CAD build for the part. Positions are in the model's coordinates, mm. A direction names the side the tool comes from. Give positions to 0.01 mm unless a question says otherwise; leave off trailing zeros. Loops run counter-clockwise (first coordinate to the right, second up) from the corner with the lowest first, then second, coordinate; pieces in that order, holes last. Notation, with made-up numbers: (2, 63.25) -> (47, 63.25) arc R9 cw to (47, 79.25) -> close; hole circle Ø1 at (88, -39). An arc over 180 degrees is marked (long way). Use one line per item in the form item = value.
```python
from build123d import *

# Parameters (mm, degrees)
F0_R     = 7.62
F1_DEPTH = 50.8
F2_R     = 1.905
F3_DEPTH = 5.715
F4_W     = 3.81
F4_H     = 7.62
F5_DEPTH = 11.431


with BuildPart() as f1:
    # F0 (on Right) → F1 (new body, symmetric)
    with BuildSketch(Plane.YZ):
        Circle(F0_R)
    extrude(amount=F1_DEPTH, both=True)

    # F2 (on Front) → F3 (join, symmetric)
    with BuildSketch(Plane.XZ):
        with BuildLine():
            Line((50.8, 3.81), (50.8, 0))
            Line((50.8, 0), (50.8, -3.81))
            Line((50.8, -3.81), (58.42, -3.81))
            ThreePointArc((58.42, -3.81), (62.23, 0), (58.42, 3.81))
            Line((58.42, 3.81), (50.8, 3.81))
        make_face()
        with Locations((58.42, 0)):
            Circle(F2_R, mode=Mode.SUBTRACT)
    extrude(amount=F3_DEPTH, both=True)

    # F4 (on face) → F5 (cut, through all)
    with BuildSketch(Plane.YZ.offset(50.8)):
        Rectangle(F4_W, F4_H)
    extrude(amount=F5_DEPTH, mode=Mode.SUBTRACT)

    # F6: F1 across plane


with BuildPart() as f1_1:
    add(f1.part)
    add(f1.part.mirror(Plane.YZ))


solid = f1_1.part
```
1. Drop flat-ended pins along their axis: P1, Ø6, axis at x = -58.42, z = 0, coming from the -Y side (3 decimals); P2, Ø5, axis at x = -3, z = 3.5, coming from the -Y side; P3, Ø6, axis at x = -8.5, y = -1, coming from the -Z side; P4, Ø1.1, axis at x = -55, y = 4.5, coming from the -Z side. Give the stop position or say it passes through.
Result sheet:
P1 = -5.715
P2 = -7.55
P3 = -7.62
P4 = -3.81
2. Tool access for faces 4 (the flat face through (-55, 4, 3.81)), 5 (the flat face through (-55, -4, -3.81)), 6 (the flat face through (55, 4, -3.81)), 7 (the flat face through (-55, -5.715, 0)), 8 (the flat face through (55, 4, 3.81)): list every direction of +Z, -Z, +X, -X, +Y, -Y with a clear straight run to the whole face (end or side of a thin tool).
Result sheet:
face_4 = +Z, -X, +Y, -Y
face_5 = -Z, -X, +Y, -Y
face_6 = -Z, +X, +Y, -Y
face_7 = +Z, -Z, -X, -Y
face_8 = +Z, +X, +Y, -Y
3. Cut at A-A, the plane y = -4.5. Write the cut outline in (x, z) (3 decimals), then the cut area to 3 significant figures.
Result sheet:
outline = (-58.42, -3.81) -> (-50.8, -3.81) -> (-50.8, -6.149) -> (50.8, -6.149) -> (50.8, -3.81) -> (58.42, -3.81) arc R3.81 ccw to (58.42, 3.81) -> (50.8, 3.81) -> (50.8, 6.149) -> (-50.8, 6.149) -> (-50.8, 3.81) -> (-58.42, 3.81) arc R3.81 ccw to start; hole circle Ø3.81 at (-58.42, 0); hole circle Ø3.81 at (58.42, 0)
area = 1,390 mm^2
4. Drill centre lines: line 1 (X direction, y = 2.8, z = 0) (3 decimals); line 2 (Y direction, x = 54, z = 2) (3 decimals); line 3 (Z direction, x = 58.42, y = 3.9) (3 decimals). Where is each one in solid material? Low to high.
Result sheet:
line_1 = -62.23 to -60.325, -56.515 to 56.515, 60.325 to 62.23
line_2 = -5.715 to -1.905, 1.905 to 5.715
line_3 = -3.81 to -1.905, 1.905 to 3.81
5. Cut at D-D, the plane z = 5.25. Write the cut outline in (x, y).
Result sheet:
outline = (-50.8, -5.52) -> (50.8, -5.52) -> (50.8, 5.52) -> (-50.8, 5.52) -> close
6. Cut at C-C, the plane y = 0. Write the cut outline in (x, z).
Result sheet:
outline = (-50.8, -7.62) -> (50.8, -7.62) -> (50.8, 7.62) -> (-50.8, 7.62) -> close
7. Mould opens along X. For faces 1 (the cylindrical face through (-62.23, -3.84, -0.08)), 2 (the flat face through (-55, 1.905, 0)), 3 (the cylindrical face through (60.237, 3.837, 0.572)) say: pulls with the +X half, pulls with the -X half, needs draft (parallel to the pull), parting line crosses it, or undercut.
Result sheet:
face_1 = pulls with the -X half
face_2 = needs draft
face_3 = undercut
8. Cut at B-B, the plane x = 12.5. Write the cut outline in (y, z), then the cut area to 3 significant figures.
Result sheet:
outline = circle Ø15.24 at (0, 0)
area = 182 mm^2
